Read the model definition and answer for the solid it produces. Units are mm, in the model's axes. Round coordinates to 2 decimals unless told otherwise and drop trailing zeros. Order: outer loops, then holes, each group sorted by start corner. A loop starts at its lowest first (then second) coordinate and runs counter-clockwise, first axis right, second up.
from build123d import *

# Parameters (mm, degrees)
SKETCH1_R           = 2.4257
BOSS_EXTRUDE1_DEPTH = 3.175


with BuildPart() as part:
    # Sketch1 → Boss-Extrude1 (new body)
    with BuildSketch(Plane(origin=(0, 0, 0), x_dir=(1, 0, 0), z_dir=(0, 1, 0))):
        Polygon((0, 0), (0, 114.3), (38.1, 114.3), (101.6, 38.1), (101.6, 0), align=None)
        with Locations(Location((15.875, 15.875, 0), (0, 0, 270))):
            Circle(SKETCH1_R, mode=Mode.SUBTRACT)
        with Locations(Location((53.975, 15.875, 0), (0, 0, 270))):
            Circle(SKETCH1_R, mode=Mode.SUBTRACT)
        with Locations(Location((92.075, 15.875, 0), (0, 0, 270))):
            Circle(SKETCH1_R, mode=Mode.SUBTRACT)
        with Locations(Location((16.891, 53.975, 0), (0, 0, 270))):
            Circle(SKETCH1_R, mode=Mode.SUBTRACT)
        with Locations(Location((16.891, 79.375, 0), (0, 0, 270))):
            Circle(SKETCH1_R, mode=Mode.SUBTRACT)
        with Locations(Location((16.891, 104.775, 0), (0, 0, 270))):
            Circle(SKETCH1_R, mode=Mode.SUBTRACT)
    extrude(amount=BOSS_EXTRUDE1_DEPTH)


solid = part.part
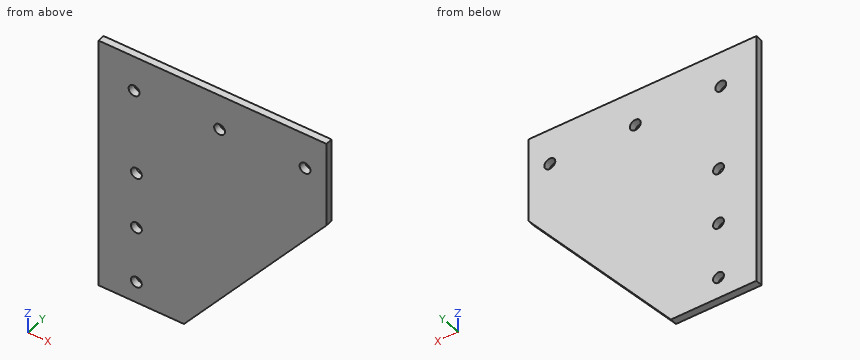
Q1. A cutting plane is placed at A-A, the plane y = 1.85. Give the vertices of the cut face in (x, z) (3 decimals).
Outcome:
outline: (0, -114.3) - (38.1, -114.3) - (101.6, -38.1) - (101.6, 0) - (0, 0) - close; hole circle Ø4.851 at (15.875, -15.875); hole circle Ø4.851 at (16.891, -104.775); hole circle Ø4.851 at (16.891, -79.375); hole circle Ø4.851 at (16.891, -53.975); hole circle Ø4.851 at (53.975, -15.875); hole circle Ø4.851 at (92.075, -15.875)
Q2. Straight lines are drawn through the part: probe 1 along Z at (x, y) = (15.5, 3.05); probe 2 along X at (y, z) = (0.75, -15); probe 3 along Z at (x, y) = (55.5, 2.65). For each, find the intervals that lie inside material, in ascending order.
Outcome:
probe 1: z = -114.3 to -106.76, -102.79 to -81.36, -77.39 to -55.96, -51.99 to -18.27, -13.48 to 0
probe 2: x = 0 to 13.61, 18.14 to 51.71, 56.24 to 89.81, 94.34 to 101.6
probe 3: z = -93.42 to -17.76, -13.99 to 0
Q3. A cutting plane is placed at B-B, the plane z = -61.5. Give the vertices of the cut face in (x, y) (3 decimals), plus the area to 3 significant figures.
Outcome:
outline: (0, 0) - (82.1, 0) - (82.1, 3.175) - (0, 3.175) - close
area: 261 mm2
Q4. Flat-ended cylindrical pins translate along their axes: pin 1 (1 mm diameter, centred on y = 2, z = -91, fed in from +X); pin 2 (1 mm diameter, centred on y = 0.5, z = -77, fed in from +X). Find the tip coordinate at first contact, or state that the pin passes through.
Outcome:
pin 1: stops at x = 57.93
pin 2: stops at x = 69.6
Q5. A cutting plane is placed at C-C, the plane x = 41. Give the vertices of the cut face in (y, z) (3 decimals).
Outcome:
outline: (0, -110.82) - (3.175, -110.82) - (3.175, 0) - (0, 0) - close
